```python
from build123d import *

# Parameters (mm, degrees)
BOSS_EXTRUDE1_DEPTH = 1
SKETCH2_R           = 0.25
CUT_EXTRUDE1_DEPTH  = 1


with BuildPart() as part:
    # Sketch1 → Boss-Extrude1 (new body)
    with BuildSketch(Plane.XY):
        with BuildLine():
            ThreePointArc((2.680014273, -3.614902972), (0, 4.5), (-2.680014273, -3.614902972))
            ThreePointArc((-2.680014273, -3.614902972), (-2.57613775, -4.314338222), (-3.275573, -4.418214744))
            ThreePointArc((-3.275573, -4.418214744), (0, 5.5), (3.275573, -4.418214744))
            ThreePointArc((3.275573, -4.418214744), (2.57613775, -4.314338222), (2.680014273, -3.614902972))
        make_face()
    extrude(amount=BOSS_EXTRUDE1_DEPTH)

    # Sketch2 → Cut-Extrude1 (cut)
    with BuildSketch(Plane.XY.offset(1)):
        with Locations((-3.090538889, -3.984232302)):
            Circle(SKETCH2_R)
        with Locations((3.090538889, -3.984232302)):
            Circle(SKETCH2_R)
    extrude(amount=-CUT_EXTRUDE1_DEPTH, mode=Mode.SUBTRACT)


solid = part.part
```
Here's how the part is built. I have some questions about the finished solid (model axes, mm). Give positions to 0.01 mm unless a question says otherwise; leave off trailing zeros. Loops run counter-clockwise (first coordinate to the right, second up) from the corner with the lowest first, then second, coordinate; pieces in that order, holes last. Notation, with made-up numbers: M 47,36.25 L 67,36.25 A32 cw 67,70.25 Z; hole C 22.25,7.5 d3. An arc over 180 degrees is marked long. Return JSON: item names as keys, results as strings.
Item 1: Imagine slicing it at B-B on x = 0. List the corners of the cut face in (y, z) for me.
A:
{"outline": "M 4.5,0 L 5.5,0 L 5.5,1 L 4.5,1 Z"}
Item 2: Imagine slicing it at C-C on z = 0.55. List the corners of the cut face in (x, y) for me, then the cut area to 3 significant figures.
A:
{"outline": "M -3.28,-4.42 A0.5 ccw -2.68,-3.61 A4.5 cw long 2.68,-3.61 A0.5 ccw 3.28,-4.42 A5.5 ccw long Z; hole C -3.09,-3.98 d0.5; hole C 3.09,-3.98 d0.5", "area": "25.4 mm^2"}
Item 3: Imagine slicing it at D-D on y = -2.5. List the corners of the cut face in (x, z) for me, then the cut area to 3 significant figures.
A:
{"outline": "M -4.9,0 L -3.74,0 L -3.74,1 L -4.9,1 Z; M 3.74,0 L 4.9,0 L 4.9,1 L 3.74,1 Z", "area": "2.31 mm^2"}
Item 4: Please list where these lines run through material, in increasing order: line 1 (Y direction, x = 0, z = 0.7); line 2 (X direction, y = -1, z = 0.9); line 3 (X direction, y = 1.25, z = 0.3).
A:
{"line 1": "y = 4.5 to 5.5", "line 2": "x = -5.41 to -4.39, 4.39 to 5.41", "line 3": "x = -5.36 to -4.32, 4.32 to 5.36"}
Item 5: Thinking about a two-plate mould opening in Y: for faces 1 (the flat face through (0, 5, 1)), 2 (the cylindrical face through (-0.193, 5.497, 0.493)), 3 (the cylindrical face through (0.158, 4.497, 0.493)), 4 (the cylindrical face through (-2.57, -4.305, 0.493)), which applies, released by +Y, released by -Y, zero draft, split by the parting line, or undercut?
A:
{"face 1": "zero draft", "face 2": "split by the parting line", "face 3": "undercut", "face 4": "undercut"}
Item 6: Imagine slicing it at A-A on y = 0. List the corners of the cut face in (x, z) for me.
A:
{"outline": "M -5.5,0 L -4.5,0 L -4.5,1 L -5.5,1 Z; M 4.5,0 L 5.5,0 L 5.5,1 L 4.5,1 Z"}
